Verification items for this drawing (mm, ordinates from the low corner). Coordinates: 2 decimals unless noted, no trailing zeros. Write each loop counter-clockwise with the first axis right and the second up, starting at its lowest first coordinate (ties: lowest second). Pieces come first, ordered by that corner, then holes. Notation, with made-up numbers: (5.5, 39) -> (24.5, 39) arc R24 cw to (24.5, 52) -> close; hole circle Ø9 at (82.25, 30.25). An arc over 180 degrees is marked (long way). One line per item, written item: value. Start each with the question number.
1) Sectioned sample at B-B on x = 153. Enter the section's corners in (y, z).
2) Scan lines: line 1 along X through (y, z) = (1.8, 90.5); line 2 along X through (y, z) = (3.6, 28); line 3 along Z through (x, y) = (114, 4.4). Record each from-to range of solid material in increasing order. Write a range as [from, to].
3) Sectioned sample at A-A on z = 90.5. Enter the section's corners in (x, y).
4) Sectioned sample at D-D on x = 73.5. Enter the section's corners in (y, z).
5) Sectioned sample at C-C on y = 5.1. Give the number of separate pieces and of enclosed holes in the cut face, plus the area to 3 significant figures.
6) Gauge pin test, flat ends, axial feed: P1, Ø8, axis at x = 29, z = 121.5, coming from the -Y side; P2, Ø1.8, axis at x = 157, y = 2, coming from the +Z side; P3, Ø1.8, axis at y = 4.5, z = 100.5, coming from the -X side; P4, Ø1.8, axis at x = 154.5, y = 4, coming from the -Z side. Record the tip position at first contact, or that the pin passes through.
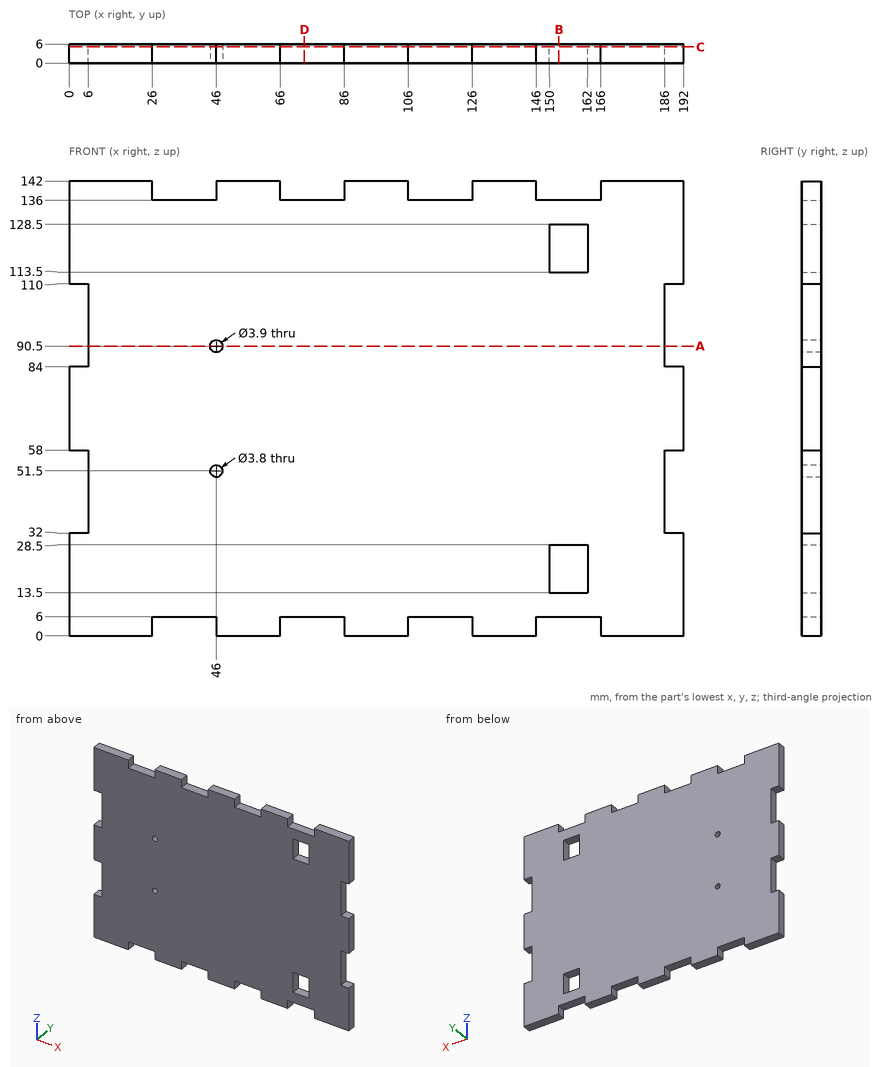
Answers:
1. outline: (0, 6) -> (6, 6) -> (6, 13.5) -> (0, 13.5) -> close; (0, 28.5) -> (6, 28.5) -> (6, 113.5) -> (0, 113.5) -> close; (0, 128.5) -> (6, 128.5) -> (6, 136) -> (0, 136) -> close
2. line 1: x = [6, 44.05], [47.95, 186]
2. line 2: x = [0, 150], [162, 192]
2. line 3: z = [6, 136]
3. outline: (6, 0) -> (44.05, 0) -> (44.05, 6) -> (6, 6) -> close; (47.95, 0) -> (186, 0) -> (186, 6) -> (47.95, 6) -> close
4. outline: (0, 6) -> (6, 6) -> (6, 136) -> (0, 136) -> close
5. separate pieces: 1
5. enclosed holes: 4
5. area: 25,300 mm2
6. P1: stops at y = 0
6. P2: stops at z = 136
6. P3: stops at x = 6
6. P4: stops at z = 6
